Input: part model. Units: mm. Frame: model coordinates. Face numbers are marked on the shaded views. A direction names the side the tool comes from. Round coordinates to 2 decimals unless told otherwise and drop trailing zeros. Order: outer loops, then holes, each group sorted by start corner. A loop starts at its lowest first (then second) coordinate and runs counter-clockwise, first axis right, second up. Notation, with made-up numbers: (81, 55.25) - (137, 55.25) arc R25 cw to (137, 79.25) - close; hole circle Ø9 at (0.25, -18.5). An arc over 180 degrees is marked (long way). One line per item, written item: value. Start each with the question number.
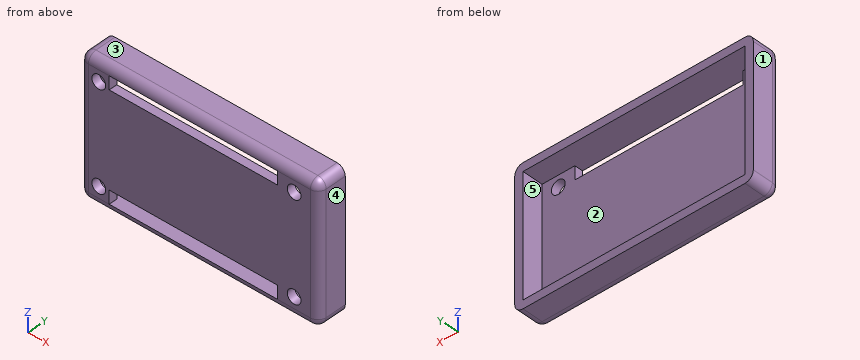
from build123d import *

# Parameters (mm, degrees)
SKETCH1_W           = 57.4
SKETCH1_H           = 33
BOSS_EXTRUDE1_DEPTH = 7
FILLET1_R           = 2
SHELL3_START        = 2
SHELL3_OUTLINE_W    = 5
SHELL3_OUTLINE_H    = 29
SHELL3_DEPTH        = 53.4
SKETCH2_R           = 1.65
CUT_EXTRUDE1_DEPTH  = 67.398493959
SKETCH3_W           = 40.5
SKETCH3_H           = 3.2
CUT_EXTRUDE2_DEPTH  = 67.398493959


# Read off the part's stored shape, not the designer's step: Shell3
with BuildPart() as part:
    # Sketch1 → Boss-Extrude1 (new body)
    with BuildSketch(Plane(origin=(0, 0, 0), x_dir=(1, 0, 0), z_dir=(0, 1, 0))):
        with Locations((28.7, 16.5)):
            Rectangle(SKETCH1_W, SKETCH1_H)
    extrude(amount=BOSS_EXTRUDE1_DEPTH)

    # Fillet1
    fillet1_edges = [part.edges().sort_by_distance(p)[0] for p in [
        (28.7, 0, -33),
        (57.4, 0, -16.5),
        (28.7, 0, 0),
        (0, 0, -16.5),
        (0, 3.5, -33),
        (57.4, 3.5, -33),
        (57.4, 3.5, 0),
        (0, 3.5, 0),
    ]]
    fillet(fillet1_edges, radius=FILLET1_R)

    # Shell3 outline → Shell3 (cut)
    with BuildSketch(Plane.YZ.offset(SHELL3_START)):
        with Locations((4.5, -16.5)):
            Rectangle(SHELL3_OUTLINE_W, SHELL3_OUTLINE_H)
    extrude(amount=SHELL3_DEPTH, mode=Mode.SUBTRACT)

    # Sketch2 → Cut-Extrude1 (cut, through all)
    with BuildSketch(Plane(origin=(0, 2, 0), x_dir=(1, 0, 0), z_dir=(0, 1, 0))):
        with Locations(Location((4.5, 28.3, 0), (0, 0, 270))):
            Circle(SKETCH2_R)
        with Locations(Location((51.5, 28.3, 0), (0, 0, 270))):
            Circle(SKETCH2_R)
        with Locations(Location((4.5, 4.7, 0), (0, 0, 270))):
            Circle(SKETCH2_R)
        with Locations(Location((51.5, 4.7, 0), (0, 0, 270))):
            Circle(SKETCH2_R)
    extrude(amount=-CUT_EXTRUDE1_DEPTH, mode=Mode.SUBTRACT)

    # Sketch3 → Cut-Extrude2 (cut, through all)
    with BuildSketch(Plane(origin=(0, 2, 0), x_dir=(1, 0, 0), z_dir=(0, 1, 0))):
        with Locations((27.25, 29.4)):
            Rectangle(SKETCH3_W, SKETCH3_H)
        with Locations((27.25, 3.6)):
            Rectangle(SKETCH3_W, SKETCH3_H)
    extrude(amount=-CUT_EXTRUDE2_DEPTH, mode=Mode.SUBTRACT)


solid = part.part
1. Section B-B (z = -9.5). Return the cut outline in (x, y).
2. Line query: line 1 (X direction, y = 6.75, z = -7); line 2 (X direction, y = 0.5, z = -4.7); line 3 (X direction, y = 0.75, z = -28.3). Output: solid intervals per line, ascending. Write a range as from..to.
3. Section A-A (x = 26). Return the cut outline in (y, z).
4. Pull-direction query (Z, two-part tool) for the marked faces 1, 2 and 3; classes: released by +Z, released by -Z, zero draft, split by the parting line, or undercut.
5. Section C-C (x = 4.5). Return the cut outline in (y, z).
6. Pin query (flat end, axial travel): pin 1 (0.6 mm diameter, centred on x = 35, y = 1, fed in from +Z); pin 2 (1 mm diameter, centred on y = 0.5, z = -30, fed in from -X); pin 3 (4.5 mm diameter, centred on x = 4.5, z = -28.3, fed in from +Y). Return the tip coordinate at first contact, or that it passes through.
7. Set-up query: the marked faces 4 and 5. Return all of +Z, -Z, +X, -X, +Y, -Y with unobstructed straight access to the full face (end or side cutting, diameter ignored); none if empty.
Solved:
1. outline: (0, 2) arc R2 ccw to (2, 0) - (55.4, 0) arc R2 ccw to (57.4, 2) - (57.4, 7) - (55.4, 7) - (55.4, 2) - (2, 2) - (2, 7) - (0, 7) - close
2. line 1: x = 0..2, 55.4..57.4
2. line 2: x = 0.68..2.85, 6.15..7, 47.5..49.85, 53.15..56.72
2. line 3: x = 0.44..2.85, 6.15..7, 47.5..49.85, 53.15..56.96
3. outline: (0, -31) arc R2 ccw to (2, -33) - (7, -33) - (7, -31) - close; (0, -27.8) - (2, -27.8) - (2, -5.2) - (0, -5.2) - close; (0, -2) - (7, -2) - (7, 0) - (2, 0) arc R2 ccw to start
4. face 1: zero draft
4. face 2: undercut
4. face 3: released by +Z
5. outline: (0, -31) arc R2 ccw to (2, -33) - (7, -33) - (7, -31) - (2, -31) - (2, -29.95) - (0, -29.95) - close; (0, -26.65) - (2, -26.65) - (2, -6.35) - (0, -6.35) - close; (0, -3.05) - (2, -3.05) - (2, -2) - (7, -2) - (7, 0) - (2, 0) arc R2 ccw to (0, -2) - close
6. pin 1: stops at z = -0.13
6. pin 2: stops at x = 0.27
6. pin 3: stops at y = 2
7. face 4: +Z, -Z, +X, +Y, -Y
7. face 5: +Y
